```python
from build123d import *

# Parameters (mm, degrees)
BOSS_EXTRUDE1_DEPTH = 4
SKETCH2_W           = 8.95
SKETCH2_H           = 19.3
SKETCH2_R           = 2.25
BOSS_EXTRUDE2_DEPTH = 4
FILLET1_R           = 10
FILLET2_R           = 4
SKETCH3_W           = 52.4
SKETCH3_H           = 19.3
SKETCH3_R           = 2
BOSS_EXTRUDE3_DEPTH = 4
FILLET3_R           = 10
SKETCH4_W           = 31
SKETCH4_H           = 20.5
CUT_EXTRUDE1_DEPTH  = 10
SKETCH5_W           = 4
SKETCH5_H           = 6
CUT_EXTRUDE2_DEPTH  = 10
FILLET4_R           = 11.55
SKETCH6_W           = 4.2
SKETCH6_H           = 4
BOSS_EXTRUDE4_DEPTH = 23.3
SKETCH7_R           = 9.5
BOSS_EXTRUDE5_DEPTH = 4
FILLET6_R           = 4


with BuildPart() as part:
    # Sketch1 → Boss-Extrude1 (new body)
    with BuildSketch(Plane(origin=(0, 0, 0), x_dir=(1, 0, 0), z_dir=(0, 1, 0))):
        Polygon((-49, 49.45), (-39, 49.45), (-39, 58.4), (0, 58.4), (0, 0), (-39, 0), (-39, 8.95), (-49, 8.95), align=None)
    extrude(amount=BOSS_EXTRUDE1_DEPTH)

    # Sketch2 → Boss-Extrude2 (add)
    # profile 1 of 2: a face of its own
    with BuildSketch(Plane.ZY.offset(39)):
        with Locations((-4.475, 13.65)):
            Rectangle(SKETCH2_W, SKETCH2_H)
        with Locations((-4.4, 18.55)):
            Circle(SKETCH2_R, mode=Mode.SUBTRACT)
        with Locations((-4.4, 8.55)):
            Circle(SKETCH2_R, mode=Mode.SUBTRACT)
    # profile 2 of 2: a face of its own
    with BuildSketch(Plane.ZY.offset(39)):
        with Locations((-53.925, 13.65)):
            Rectangle(SKETCH2_W, SKETCH2_H)
        with Locations((-53.45, 18.55)):
            Circle(SKETCH2_R, mode=Mode.SUBTRACT)
        with Locations((-53.45, 8.55)):
            Circle(SKETCH2_R, mode=Mode.SUBTRACT)
    extrude(amount=-BOSS_EXTRUDE2_DEPTH)

    # Fillet1
    # the kernel refuses this fillet: 10 mm, written as the material it adds along each edge
    with BuildSketch(Plane(origin=(-39, 0, -49.45), x_dir=(-1, 0, 0), z_dir=(0, 1, 0))) as fillet1_piece_1:
        with BuildLine():
            CenterArc((9.944722218, -10), FILLET1_R, 90, 83.97283344)
            Line((0, -8.95), (0, 0))
            Line((0, 0), (9.944722218, 0))
        make_face()
    extrude(amount=4)
    with BuildSketch(Plane(origin=(-39, 0, -8.95), x_dir=(0, 0, 1), z_dir=(0, 1, 0))) as fillet1_piece_2:
        with BuildLine():
            CenterArc((10, -9.944722218), FILLET1_R, 96.02716656, 83.97283344)
            Line((0, -9.944722218), (0, 0))
            Line((0, 0), (8.95, 0))
        make_face()
    extrude(amount=4)

    # Fillet2
    fillet2_edges = [part.edges().sort_by_distance(p)[0] for p in [
        (-37, 23.3, 0),
        (-37, 23.3, -58.4),
    ]]
    fillet(fillet2_edges, radius=FILLET2_R)

    # Sketch3 → Boss-Extrude3 (add)
    with BuildSketch(Plane(origin=(0, 0, 0), x_dir=(0, 0, -1), z_dir=(1, 0, 0))):
        with Locations((26.2, 13.65)):
            Rectangle(SKETCH3_W, SKETCH3_H)
        with Locations((18.45, 13.55)):
            Circle(SKETCH3_R, mode=Mode.SUBTRACT)
    extrude(amount=-BOSS_EXTRUDE3_DEPTH)

    # Fillet3
    fillet3_edges = [part.edges().sort_by_distance(p)[0] for p in [
        (-2, 23.3, 0),
    ]]
    fillet(fillet3_edges, radius=FILLET3_R)

    # Sketch4 → Cut-Extrude1 (cut)
    with BuildSketch(Plane(origin=(0, 4, 0), x_dir=(1, 0, 0), z_dir=(0, 1, 0))):
        with Locations((-19.5, 48.15)):
            Rectangle(SKETCH4_W, SKETCH4_H)
    extrude(amount=-CUT_EXTRUDE1_DEPTH, mode=Mode.SUBTRACT)

    # Sketch5 → Cut-Extrude2 (cut)
    with BuildSketch(Plane(origin=(0, 4, 0), x_dir=(1, 0, 0), z_dir=(0, 1, 0))):
        with Locations((-2, 55.4)):
            Rectangle(SKETCH5_W, SKETCH5_H)
    extrude(amount=-CUT_EXTRUDE2_DEPTH, mode=Mode.SUBTRACT)

    # Fillet4
    fillet4_edges = [part.edges().sort_by_distance(p)[0] for p in [
        (-35, 2, -37.9),
    ]]
    fillet(fillet4_edges, radius=FILLET4_R)

    # Sketch6 → Boss-Extrude4 (add)
    with BuildSketch(Plane.XZ):
        with Locations((2.1, -50.4)):
            Rectangle(SKETCH6_W, SKETCH6_H)
    extrude(amount=-BOSS_EXTRUDE4_DEPTH)

    # Sketch7 → Boss-Extrude5 (add)
    with BuildSketch(Plane(origin=(4.2, 0, 0), x_dir=(0, 0, -1), z_dir=(1, 0, 0))):
        with BuildLine():
            Line((48.4, 0), (48.4, 23.3))
            Line((48.4, 23.3), (62.9, 23.3))
            Line((62.9, 23.3), (66.1, 26.5))
            Line((66.1, 26.5), (76, 26.5))
            ThreePointArc((76, 26.5), (88.6, 13.9), (76, 1.3))
            Line((76, 1.3), (64.2, 1.3))
            Line((64.2, 1.3), (62.9, 0))
            Line((62.9, 0), (48.4, 0))
        make_face()
        with Locations((76, 13.9)):
            Circle(SKETCH7_R, mode=Mode.SUBTRACT)
    extrude(amount=BOSS_EXTRUDE5_DEPTH)

    # Fillet6
    fillet6_edges = [part.edges().sort_by_distance(p)[0] for p in [
        (4.2, 11.65, -52.4),
        (0, 11.65, -48.4),
        (8.2, 11.65, -48.4),
        (-4, 11.65, -52.4),
    ]]
    fillet(fillet6_edges, radius=FILLET6_R)


solid = part.part
```
Geometry check sheet. Reference: the model listing, model coordinates, mm. A direction names the side the tool comes from. Coordinates: 2 decimals unless noted, no trailing zeros. Write each loop counter-clockwise with the first axis right and the second up, starting at its lowest first coordinate (ties: lowest second). Pieces come first, ordered by that corner, then holes. Notation, with made-up numbers: M 88.5,35.5 L 115.5,35.5 A23 ccw 115.5,72.5 Z; hole C 59.5,47.25 d3. An arc over 180 degrees is marked long. Use one line per item in the form item = value. Start each with the question number.
1) Section check D-D on x = -21. Enter the section's corners in (y, z), and give its area (3 significant figures).
2) Set-up check for faces 1 (the flat face through (-37, 10, -58.4)), 2 (the flat face through (-37, 14, -49.45)), 3 (the flat face through (6, 1.3, -70)), 4 (the cylindrical face through (-37.03, 17.69, -51.37)), 5 (the cylindrical face through (-31.706, 1.972, -41.373)): record each of +Z, -Z, +X, -X, +Y, -Y from which the full face is reachable in a straight line by a thin tool's end or side.
3) Release check for a two-part mould opening along Z. For faces 6 (the flat face through (-37, 23.3, -7)), 7 (the cylindrical face through (-36.972, 22.097, -57.259)), 8 (the flat face through (-37, 14, -8.95)) record: pulls with the +Z half, pulls with the -Z half, needs draft (parallel to the pull), parting line crosses it, or undercut.
4) Section check B-B on y = 8.55. State how many separate pieces and enclosed holes the cut face has, and give its area (3 significant figures).
5) Thickness scan on probe 1 along Y at (x, z) = (-37.35, -4.4); probe 2 along Z at (x, y) = (-36, 15.25); probe 3 along Y at (x, z) = (-1.85, -18.45). Record the ranges inside material, lowest first. Write a range as from..to.
6) Section check C-C on z = -53.45. Enter the section's corners in (x, y), and give its area (3 significant figures).
7) Section check A-A on z = -18.45. Enter the section's corners in (x, y), and give its area (3 significant figures).
8) Go/stop test with flat-tipped pins: pin 1 Ø12 at (x, z) = (-22, -28.5) entering from +Y; pin 2 Ø1.5 at (y, z) = (9.5, -43.5) entering from -X; pin 3 Ø3.5 at (x, z) = (3.5, -40.5) entering from +Y; pin 4 Ø1.2 at (x, y) = (-11.5, 1.5) entering from -Z. Record where each tip stops, or that it passes through.
Responses:
q1.outline = M 0,-37.9 L 4,-37.9 L 4,0 L 0,0 Z
q1.area = 152 mm2
q2.face_1 = -Z, -X, +Y, -Y
q2.face_2 = -X, +Y
q2.face_3 = -Z, +X, -X, -Y
q2.face_4 = -X
q2.face_5 = -Z, +Y, -Y
q3.face_6 = needs draft
q3.face_7 = pulls with the -Z half
q3.face_8 = undercut
q4.separate_pieces = 6
q4.enclosed_holes = 0
q4.area = 355 mm2
q5.probe_1 = 0..6.3, 10.8..16.3, 20.8..23.3
q5.probe_2 = -58.4..-49.45, -8.95..0
q5.probe_3 = 0..11.55, 15.55..23.3
q6.outline = M -40.94,0 L -35,0 L -35,6.3 L -39,6.3 L -39,4 L -40.94,4 Z; M -39,10.8 L -35,10.8 L -35,16.3 L -39,16.3 Z; M -39,20.8 L -35,20.8 L -35,23.3 L -39,23.3 Z; M 2.9,0 L 8.2,0 L 8.2,23.3 L 2.9,23.3 Z
q6.area = 188 mm2
q7.outline = M -49,0 L 0,0 L 0,11.55 L -4,11.55 L -4,4 L -49,4 Z; M -4,15.55 L 0,15.55 L 0,23.3 L -4,23.3 Z
q7.area = 257 mm2
q8.pin_1 = 4
q8.pin_2 = -4
q8.pin_3 = through
q8.pin_4 = -37.9
